```python
from build123d import *

# Parameters (mm, degrees)
CROQUIS1_R              = 13.3
SALIENTE_EXTRUIR1_DEPTH = 30
CROQUIS2_R              = 30
CROQUIS2_R_2            = 2.25
SALIENTE_EXTRUIR2_DEPTH = 8


with BuildPart() as part:
    # Croquis1 → Saliente-Extruir1 (new body)
    with BuildSketch(Plane.XY):
        Circle(CROQUIS1_R)
    extrude(amount=-SALIENTE_EXTRUIR1_DEPTH)

    # Croquis2 → Saliente-Extruir2 (add)
    with BuildSketch(Plane.XY):
        Circle(CROQUIS2_R)
        with Locations((0, 22.5)):
            Circle(CROQUIS2_R_2, mode=Mode.SUBTRACT)
        with Locations((22.5, 0)):
            Circle(CROQUIS2_R_2, mode=Mode.SUBTRACT)
        with Locations((0, -22.5)):
            Circle(CROQUIS2_R_2, mode=Mode.SUBTRACT)
        with Locations((-22.5, 0)):
            Circle(CROQUIS2_R_2, mode=Mode.SUBTRACT)
    extrude(amount=SALIENTE_EXTRUIR2_DEPTH)


solid = part.part
```
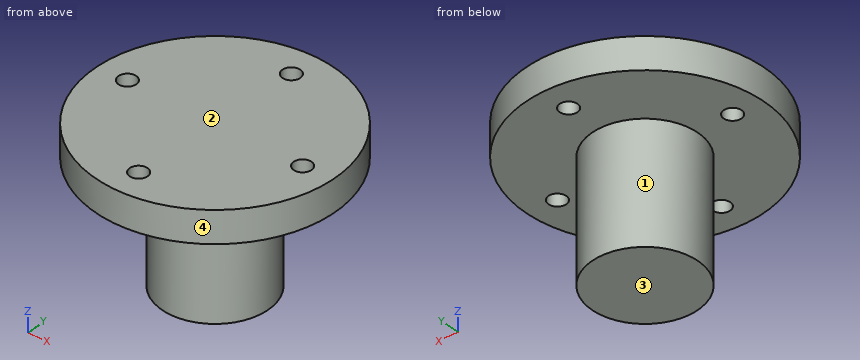
For this review, take the finished solid that the model builds, in its own axes (mm). Face numbers are marked on the shaded views. A direction names the side the tool comes from. Round coordinates to 2 decimals unless told otherwise and drop trailing zeros. Loops run counter-clockwise (first coordinate to the right, second up) from the corner with the lowest first, then second, coordinate; pieces in that order, holes last.
Q1. Add section C-C on y = -23.5. Write out the cut boundary in (x, z).
Result sheet:
outline: (-18.65, 0) - (-2.02, 0) - (-2.02, 8) - (-18.65, 8) - close; (2.02, 0) - (18.65, 0) - (18.65, 8) - (2.02, 8) - close
Q2. Mouldability with a two-part tool opening along Y and no side actions: class the marked faces 3 and 4 as +Y half, -Y half, draft (parallel to the pull), parting line (faces both ways), or undercut.
Result sheet:
face 3: draft
face 4: parting line
Q3. Add section D-D on x = -22.5. Write out the cut boundary in (y, z), plus the area to 3 significant figures.
Result sheet:
outline: (-19.84, 0) - (-2.25, 0) - (-2.25, 8) - (-19.84, 8) - close; (2.25, 0) - (19.84, 0) - (19.84, 8) - (2.25, 8) - close
area: 281 mm2
Q4. Insertion check: pin 1 Ø12 at (y, z) = (-24, 1.5) entering from -X; pin 2 Ø10 at (y, z) = (-4.5, -17.5) entering from -X; pin 3 Ø1.5 at (x, z) = (0, -10.5) entering from +Y. Each pin has a flat end and moves straight along its axis. Give the tip position at first contact, or say it passes through.
Result sheet:
pin 1: stops at x = -24
pin 2: stops at x = -13.3
pin 3: stops at y = 13.3
Q5. Machinability: for the marked faces 1 and 2, which of the approach directions +Z, -Z, +X, -X, +Y, -Y give a long, thin tool a straight path to every point of the face, cutting with its end or side? Answer none if there is none.
Result sheet:
face 1: -Z
face 2: +Z, +X, -X, +Y, -Y
Q6. To check wall thickness, follow line 1 along Y through (x, z) = (0, 2.25); line 2 along Z through (x, y) = (16.5, 6); line 3 along X through (y, z) = (22, 2). State the ranges of each line that lie inside material, in increasing order.
Result sheet:
line 1: y = -30 to -24.75, -20.25 to 20.25, 24.75 to 30
line 2: z = 0 to 8
line 3: x = -20.4 to -2.19, 2.19 to 20.4
Q7. Add section A-A on x = 0. Write out the cut boundary in (y, z).
Result sheet:
outline: (-30, 0) - (-24.75, 0) - (-24.75, 8) - (-30, 8) - close; (-20.25, 0) - (-13.3, 0) - (-13.3, -30) - (13.3, -30) - (13.3, 0) - (20.25, 0) - (20.25, 8) - (-20.25, 8) - close; (24.75, 0) - (30, 0) - (30, 8) - (24.75, 8) - close
